Geometry check sheet. Reference: drawing and pictorial views, mm from the part's lowest x, y, z. Give positions to 0.01 mm unless a question says otherwise; leave off trailing zeros. Write each loop counter-clockwise with the first axis right and the second up, starting at its lowest first coordinate (ties: lowest second). Pieces come first, ordered by that corner, then holes. Notation, with made-up numbers: (-40, 84) -> (1, 84) arc R9 cw to (1, 91) -> close; hole circle Ø2 at (29, 68.25). An arc over 180 degrees is marked (long way). Return JSON: item names as keys, results as strings.
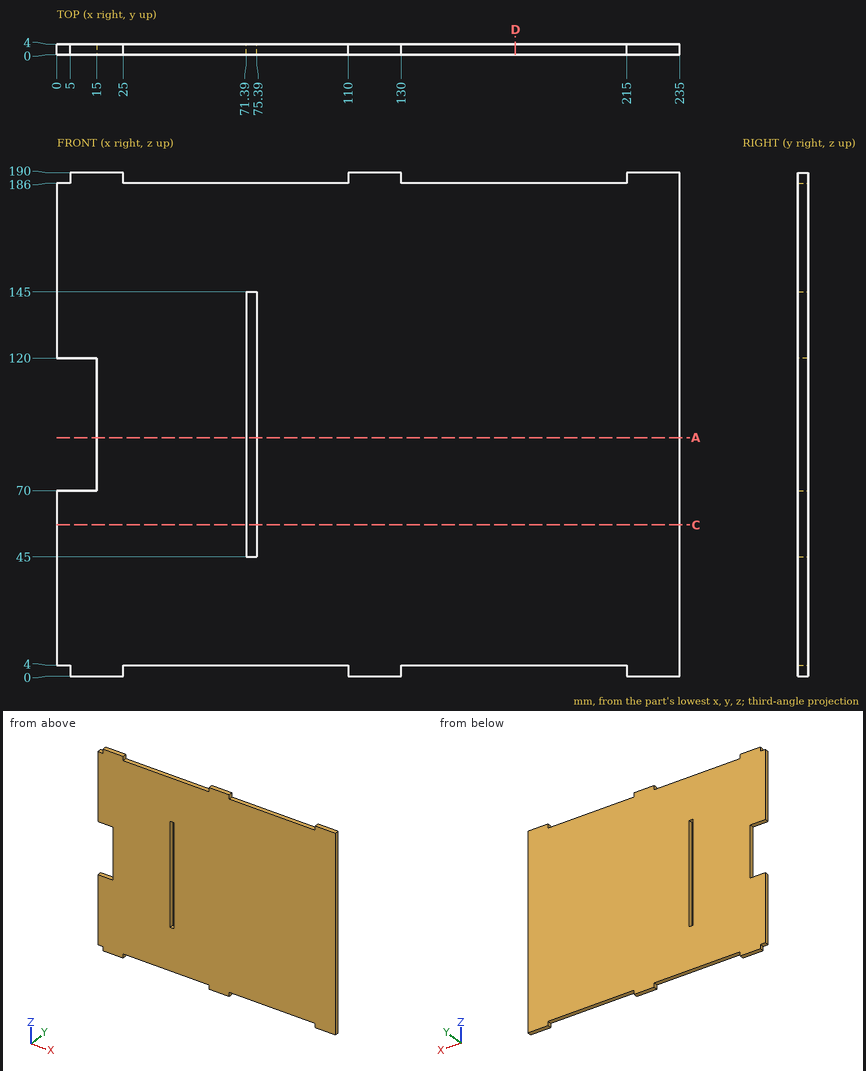
(1) Cross-section at A-A on z = 90. Enter the section's corners in (x, y).
Reply:
{"outline": "(15, 0) -> (71.39, 0) -> (71.39, 4) -> (15, 4) -> close; (75.39, 0) -> (235, 0) -> (235, 4) -> (75.39, 4) -> close"}
(2) Thickness scan on L1, parallel to X at y = 0.75, z = 111; L2, parallel to X at y = 0.9, z = 62.5; L3, parallel to Z at x = 163, y = 2.7. Record the ranges inside material, lowest first.
Reply:
{"L1": "15 to 71.39, 75.39 to 235", "L2": "0 to 71.39, 75.39 to 235", "L3": "4 to 186"}
(3) Depth check by flat-ended pin: pin 1 Ø2 at (x, y) = (160, 2) entering from +Z; pin 2 Ø1.2 at (y, z) = (1.5, 188.5) entering from -X; pin 3 Ø2 at (y, z) = (3, 74) entering from -X. Enter the tip coordinate at first touch or a pass-through.
Reply:
{"pin 1": "z = 186", "pin 2": "x = 5", "pin 3": "x = 15"}
(4) Cross-section at D-D on x = 173. Enter the section's corners in (y, z).
Reply:
{"outline": "(0, 4) -> (4, 4) -> (4, 186) -> (0, 186) -> close"}
(5) Cross-section at C-C on z = 57. Enter the section's corners in (x, y), then the cut area to 3 significant figures.
Reply:
{"outline": "(0, 0) -> (71.39, 0) -> (71.39, 4) -> (0, 4) -> close; (75.39, 0) -> (235, 0) -> (235, 4) -> (75.39, 4) -> close", "area": "924 mm^2"}
